Read the model definition and answer for the solid it produces. Units are mm, in the model's axes. Face numbers are marked on the shaded views. Coordinates: 2 decimals unless noted, no trailing zeros. Order: outer loops, then holes, each group sorted by start corner. A loop starts at its lowest first (then second) coordinate and runs counter-clockwise, first axis right, second up. Notation, with made-up numbers: (-26.5, -31) -> (-1.5, -31) arc R26 ccw to (-1.5, -15) -> close; hole circle Ø9 at (-23.75, 12.25). An arc over 180 degrees is marked (long way). Use CSV: the item, a comma, the result in double quotes.
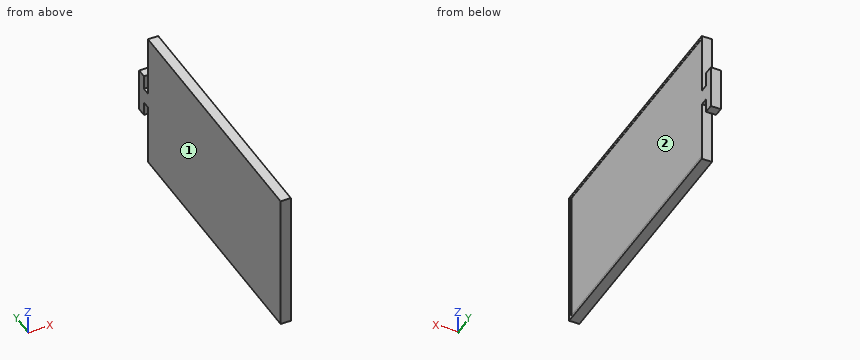
Autodesk Inventor part; units mm, degrees
ref_plane "YZ Plane" through (0, 0, 0) normal (1, 0, 0) x (0, 1, 0)
ref_plane "XZ Plane" through (0, 0, 0) normal (0, 1, 0) x (-1, 0, 0)
ref_plane "XY Plane" through (0, 0, 0) normal (0, 0, 1) x (1, 0, 0)
sketch "Sketch1" plane through (0, 0, 0) normal (1, 0, 0) x (0, 1, 0)
  line L0 (82.3549, 41.969) -> (-47.6451, 41.969)
  line L1 (-47.6451, 41.969) -> (-47.6451, -28.031)
  line L2 (-47.6451, -28.031) -> (82.3549, -28.031)
  line L3 (82.3549, -28.031) -> (82.3549, 41.969)
  point P0 (0, 0)
  dimension "d0" = 130
  dimension "d1" = 70
extrude "Extrusion1" add sketch "Sketch1" along normal blind 5
sketch "Sketch13" plane through (5, 0, 0) normal (1, 0, 0) x (0, 0, -1)
  line L0 (-41.969, -47.6451) -> (28.031, -47.6451)
  line L1 (28.031, 82.3549) -> (-41.969, 82.3549)
  line L2 (28.031, -47.6451) -> (26.531, -47.6451)
  line L3 (26.531, -47.6451) -> (26.531, 82.3549)
  line L4 (26.531, 82.3549) -> (28.031, 82.3549)
  line L5 (28.031, 82.3549) -> (28.031, -47.6451)
  line L6 (-41.969, 82.3549) -> (-41.969, -47.6451)
  line L7 (28.031, 82.3549) -> (-41.969, 82.3549)
  line L8 (-41.969, -47.6451) -> (-40.469, -47.6451)
  line L9 (-40.469, -47.6451) -> (-40.469, 82.3549)
  line L10 (-40.469, 82.3549) -> (-41.969, 82.3549)
  line L11 (-41.969, 82.3549) -> (-41.969, -47.6451)
  line L12 (28.031, -47.6451) -> (-41.969, -47.6451)
  line L13 (-41.969, -47.6451) -> (-41.969, -45.6451)
  line L14 (-41.969, -45.6451) -> (28.031, -45.6451)
  line L15 (28.031, -45.6451) -> (28.031, -47.6451)
  point P0 (0, 0)
  point P1 (10.031, 62.3549)
  point P2 (-5.969, 62.3549)
  point P3 (26.531, -45.6451)
  point P4 (-40.469, -45.6451)
  point P5 (18.031, 62.3549)
  dimension "d42" = 1.5
  dimension "d43" = 1.5
  dimension "d44" = 2
extrude "Extrusion7" add sketch "Sketch13" along normal blind 0.1 contours L6 L14 L9 L0 | L9 L14 L3 L0 | L6 L1 L9 L14 | L3 L14 L5 L0 | L3 L1 L5 L14
sketch "Sketch14" plane through (0, 82.3549, 41.969) normal (0, 1, 0) x (1, 0, 0)
  line L0 (5, 1.5) -> (5, 68.5)
  line L1 (5, 68.5) -> (5, 46.05)
  line L2 (5, 1.5) -> (5, 23.95)
  line L3 (5, 46.05) -> (0, 46.05)
  line L4 (5, 29.05) -> (5, 46.05)
  line L5 (0, 70) -> (0, 0)
  line L6 (5, 46.05) -> (0, 46.05)
  line L7 (0, 46.05) -> (0, 23.95)
  line L8 (0, 23.95) -> (5, 23.95)
  line L9 (5, 23.95) -> (5, 46.05)
  point P0 (0, 41.969)
  dimension "d47" = 22.45
  dimension "d48" = 22.45
extrude "Extrusion8" add sketch "Sketch14" along normal blind 8.65
sketch "Sketch15" plane through (5, 0, 0) normal (1, 0, 0) x (0, 0, -1)
  line L0 (28.031, 82.3549) -> (4.081, 82.3549)
  line L1 (4.081, 82.3549) -> (-3.069, 82.3549)
  line L2 (-3.069, 82.3549) -> (-3.069, 86.3549)
  line L3 (-3.069, 86.3549) -> (4.081, 86.3549)
  line L4 (4.081, 86.3549) -> (4.081, 82.3549)
  line L5 (-18.019, 82.3549) -> (-40.469, 82.3549)
  line L6 (-18.019, 82.3549) -> (-10.869, 82.3549)
  line L7 (-10.869, 82.3549) -> (-10.869, 86.3549)
  line L8 (-10.869, 86.3549) -> (-18.019, 86.3549)
  line L9 (-18.019, 86.3549) -> (-18.019, 82.3549)
  point P0 (0, 0)
  dimension "d51" = 7.15
  dimension "d52" = 7.15
  dimension "d55" = 4
extrude "Extrusion9" cut sketch "Sketch15" against normal blind 8.65
properties part number "baseplateproto1"
Item 1: Each of these flat-tipped pins is pushed along its axis until it touches: P1, Ø2.5, axis at x = 2.5, y = 88, coming from the +Z side; P2, Ø1.2, axis at x = 3, y = 85, coming from the -Z side; P3, Ø2.5, axis at x = 2, z = -11.5, coming from the +Y side. Where does it stop, or does it pass through?
Return value:
P1,"stops at z = 18.02"
P2,"stops at z = 3.07"
P3,"stops at y = 82.35"
Item 2: The mould has two halves that part along Z. Classify the marked faces 1 and 2: +Z half, -Z half, draft (parallel to the pull), parting line (faces both ways), or undercut.
Return value:
face 1,"draft"
face 2,"undercut"
Item 3: Find section C-C, the plane y = 19. Give the vertices of the cut face in (x, z).
Return value:
outline,"(0, -28.03) -> (5.1, -28.03) -> (5.1, -26.53) -> (5, -26.53) -> (5, 40.47) -> (5.1, 40.47) -> (5.1, 41.97) -> (0, 41.97) -> close"
Item 4: Find section A-A, the plane z = 0.5. Give the vertices of the cut face in (x, y), then the cut area to 3 significant figures.
Return value:
outline,"(0, -47.65) -> (5.1, -47.65) -> (5.1, -45.65) -> (5, -45.65) -> (5, 82.35) -> (0, 82.35) -> close; (0, 86.35) -> (5, 86.35) -> (5, 91) -> (0, 91) -> close"
area,"673 mm^2"
Item 5: Find section B-B, the plane x = 4.2. Give the vertices of the cut face in (y, z), then the cut area to 3 significant figures.
Return value:
outline,"(-47.65, -28.03) -> (82.35, -28.03) -> (82.35, 3.07) -> (86.35, 3.07) -> (86.35, -4.08) -> (91, -4.08) -> (91, 18.02) -> (86.35, 18.02) -> (86.35, 10.87) -> (82.35, 10.87) -> (82.35, 41.97) -> (-47.65, 41.97) -> close"
area,"9,230 mm^2"
Item 6: Straight lines are drawn through the part: line 1 along X through (y, z) = (-33, -10.5); line 2 along Y through (x, z) = (1.35, 22). For each, find the intervals that lie inside material, in ascending order.
Return value:
line 1,"x = 0 to 5"
line 2,"y = -47.65 to 82.35"
Item 7: Find section D-D, the plane z = 31. Give the vertices of the cut face in (x, y).
Return value:
outline,"(0, -47.65) -> (5.1, -47.65) -> (5.1, -45.65) -> (5, -45.65) -> (5, 82.35) -> (0, 82.35) -> close"
